Source: three-view drawing plus pictorial views. Frame: mm from the lowest corner of the part. A direction names the side the tool comes from. Give positions to 0.01 mm unless a question says otherwise; leave off trailing zeros. Write each loop counter-clockwise with the first axis right and the second up, starting at its lowest first coordinate (ties: lowest second). Pieces come first, ordered by that corner, then holes.
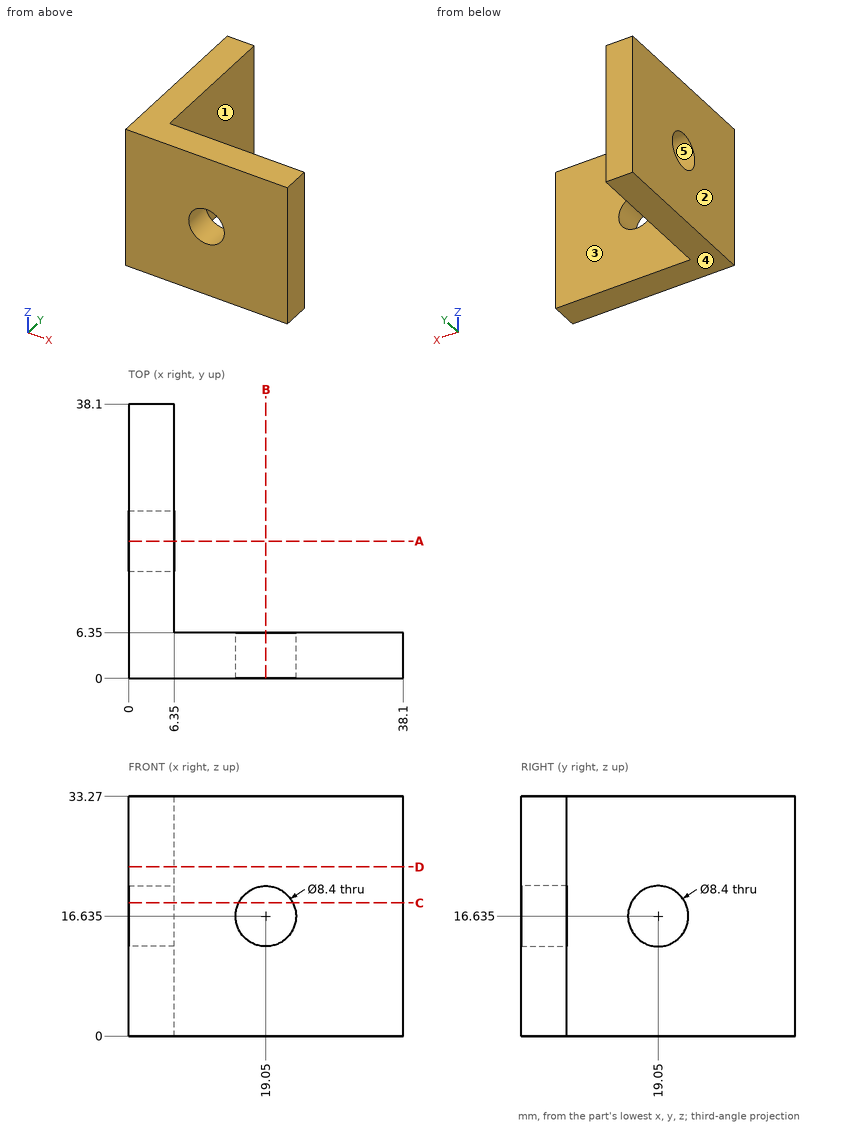
Q1. Pin query (flat end, axial travel): P1, Ø12, axis at x = 31, y = 10, coming from the -Z side; P2, Ø9.5, axis at y = 17.5, z = 21, coming from the +X side. Return the tip coordinate at first contact, or that it passes through.
Filled sheet:
P1: stops at z = 0
P2: stops at x = 6.35
Q2. Ray query, line 1 along Z through (x, y) = (3, 19); line 2 along X through (y, z) = (3, 16.5); line 3 along Y through (x, z) = (32.5, 16). Return the intervals inside material, ascending.
Filled sheet:
line 1: z = 0 to 12.44, 20.83 to 33.27
line 2: x = 0 to 14.85, 23.25 to 38.1
line 3: y = 0 to 6.35
Q3. Section D-D on z = 23.5. Output: boundary loops of the cut face in (x, y), plus the area to 3 significant figures.
Filled sheet:
outline: (0, 0) - (38.1, 0) - (38.1, 6.35) - (6.35, 6.35) - (6.35, 38.1) - (0, 38.1) - close
area: 444 mm2
Q4. Pull-direction query (Z, two-part tool) for the marked faces 3, 4 and 5; classes: released by +Z, released by -Z, zero draft, split by the parting line, or undercut.
Filled sheet:
face 3: zero draft
face 4: released by -Z
face 5: undercut
Q5. Section A-A on y = 19.05. Output: boundary loops of the cut face in (x, z) (3 decimals), plus the area to 3 significant figures.
Filled sheet:
outline: (0, 0) - (6.35, 0) - (6.35, 12.435) - (0, 12.435) - close; (0, 20.835) - (6.35, 20.835) - (6.35, 33.27) - (0, 33.27) - close
area: 158 mm2
Q6. Section C-C on z = 18.5. Output: boundary loops of the cut face in (x, y).
Filled sheet:
outline: (0, 0) - (15.29, 0) - (15.29, 6.35) - (6.35, 6.35) - (6.35, 15.29) - (0, 15.29) - close; (0, 22.81) - (6.35, 22.81) - (6.35, 38.1) - (0, 38.1) - close; (22.81, 0) - (38.1, 0) - (38.1, 6.35) - (22.81, 6.35) - close
Q7. Access query for the marked faces 1 and 2. Directions: +Z, -Z, +X, -X, +Y, -Y. A direction counts if a zero-diameter tool reaches every point of the face in a straight line with its end or side. Return the directions, or none.
Filled sheet:
face 1: +Z, -Z, +X, +Y
face 2: +Z, -Z, -X, +Y, -Y
